from build123d import *

# Parameters (mm, degrees)
SALIENTE_EXTRUIR1_DEPTH = 159.5
REDONDEO1_R             = 0.5
REDONDEO2_R             = 1
REDONDEO3_R             = 1.5
REDONDEO4_R             = 1.5


with BuildPart() as part:
    # Croquis1 → Saliente-Extruir1 (new body)
    with BuildSketch(Plane(origin=(0, 0, 0), x_dir=(1, 0, 0), z_dir=(0, 1, 0))):
        Polygon((0, 0), (0, 31.5), (-31, 31.5), (-31, 30), (-1.5, 30), (-1.5, 18.5), (-3.8, 18.5), (-3.8, 19.3), (-4.7, 19.3), (-4.7, 17.5), (-1.5, 17.5), (-1.5, 12.5), (-4.7, 12.5), (-4.7, 10.7), (-3.8, 10.7), (-3.8, 11.5), (-1.5, 11.5), (-1.5, 0), align=None)
    extrude(amount=SALIENTE_EXTRUIR1_DEPTH)

    # Redondeo1
    redondeo1_edges = [part.edges().sort_by_distance(p)[0] for p in [
        (-4.7, 79.75, -10.7),
        (-4.7, 79.75, -19.3),
    ]]
    fillet(redondeo1_edges, radius=REDONDEO1_R)

    # Redondeo2
    redondeo2_edges = [part.edges().sort_by_distance(p)[0] for p in [
        (-1.5, 79.75, -12.5),
        (-1.5, 79.75, -17.5),
    ]]
    fillet(redondeo2_edges, radius=REDONDEO2_R)

    # Redondeo3
    redondeo3_edges = [part.edges().sort_by_distance(p)[0] for p in [
        (-1.5, 79.75, -30),
    ]]
    fillet(redondeo3_edges, radius=REDONDEO3_R)

    # Redondeo4
    redondeo4_edges = [part.edges().sort_by_distance(p)[0] for p in [
        (0, 79.75, -31.5),
    ]]
    fillet(redondeo4_edges, radius=REDONDEO4_R)


solid = part.part
Source: CAD feature listing. Evaluate the final solid. Frame: model axes, mm. A direction names the side the tool comes from. Give positions to 0.01 mm unless a question says otherwise; leave off trailing zeros. Write each loop counter-clockwise with the first axis right and the second up, starting at its lowest first coordinate (ties: lowest second). Pieces come first, ordered by that corner, then holes. Notation, with made-up numbers: (72, 74) - (85, 74) arc R27 cw to (85, 101) - close; hole circle Ø1 at (66, 9). An arc over 180 degrees is marked (long way). Write item = value, one per line. Start each with the question number.
Q1. Cut plane B-B, the plane z = -21. Return loops of the section in (x, y), then the cut area to 3 significant figures.
Q2. Reachability of faces 1 (the flat face through (0, 79, -15)), 2 (the flat face through (-1.5, 79, -15)) from +Z, -Z, +X, -X, +Y, -Y: full face, straight path, thin tool, end or side. Return the list, or none.
Q3. Cut plane C-C, the plane x = -19. Return loops of the section in (y, z), then the cut area to 3 significant figures.
Q4. Material intervals for probe 1 along Z at (x, y) = (-27, 44); probe 2 along X at (y, z) = (151, -6); probe 3 along X at (y, z) = (135, -19), sorted ascending.
Q5. Cut plane A-A, the plane y = 30. Return loops of the section in (x, z), then the cut area to 3 significant figures.
Q6. Pin query (flat end, axial travel): pin 1 Ø3.5 at (y, z) = (90, -14.5) entering from -X; pin 2 Ø12 at (x, y) = (-14, 35) entering from +Z; pin 3 Ø3.5 at (y, z) = (42, -8) entering from -X; pin 4 Ø3 at (x, z) = (-5.5, -13) entering from -Y. Return the tip coordinate at first contact, or that it passes through.
Computed values:
q1.outline = (-1.5, 0) - (0, 0) - (0, 159.5) - (-1.5, 159.5) - close
q1.area = 239 mm²
q2.face_1 = +Z, -Z, +X, +Y, -Y
q2.face_2 = -X, +Y, -Y
q3.outline = (0, -31.5) - (159.5, -31.5) - (159.5, -30) - (0, -30) - close
q3.area = 239 mm²
q4.probe_1 = -31.5 to -30
q4.probe_2 = -1.5 to 0
q4.probe_3 = -4.66 to -3.8, -1.5 to 0
q5.outline = (-31, -31.5) - (-1.5, -31.5) arc R1.5 ccw to (0, -30) - (0, 0) - (-1.5, 0) - (-1.5, -11.5) - (-3.8, -11.5) - (-3.8, -10.7) - (-4.2, -10.7) arc R0.5 ccw to (-4.7, -11.2) - (-4.7, -12.5) - (-2.5, -12.5) arc R1 cw to (-1.5, -13.5) - (-1.5, -16.5) arc R1 cw to (-2.5, -17.5) - (-4.7, -17.5) - (-4.7, -18.8) arc R0.5 ccw to (-4.2, -19.3) - (-3.8, -19.3) - (-3.8, -18.5) - (-1.5, -18.5) - (-1.5, -28.5) arc R1.5 cw to (-3, -30) - (-31, -30) - close
q5.area = 99.7 mm²
q6.pin_1 = -1.84
q6.pin_2 = -30
q6.pin_3 = -1.5
q6.pin_4 = 0
